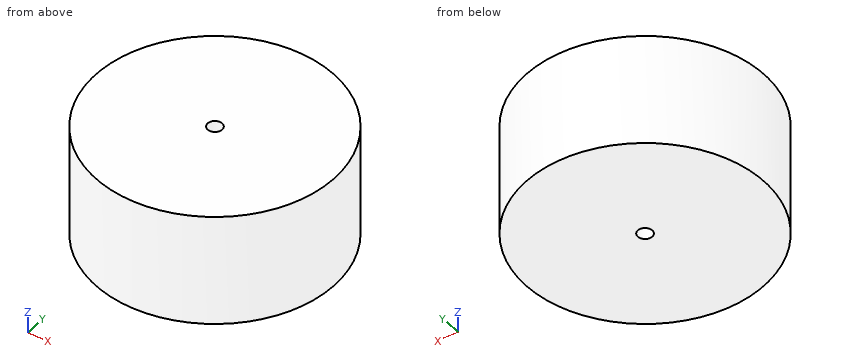
from build123d import *

# Parameters (mm, degrees)
CYLINDER_R     = 3.9
CYLINDER_DEPTH = 60
SKETCH_R       = 64
PAD_DEPTH      = 60


with BuildPart() as cylinder:
    # Cylinder → Cylinder (new body)
    with BuildSketch(Plane.XY):
        Circle(CYLINDER_R)
    extrude(amount=CYLINDER_DEPTH)


with BuildPart() as cut:
    # Sketch → Pad (new body)
    with BuildSketch(Plane.XY):
        Circle(SKETCH_R)
    extrude(amount=PAD_DEPTH)

    # Cut: cut Cylinder
    add(cylinder.part, mode=Mode.SUBTRACT)


with BuildPart() as cut_1:
    # Cut placement: moved
    add(cut.part.moved(Location((-90, -440, 0))))


solid = cut_1.part
Build history of the part. All positions in model axes, mm. Give positions to 0.01 mm unless a question says otherwise; leave off trailing zeros. Loops run counter-clockwise (first coordinate to the right, second up) from the corner with the lowest first, then second, coordinate; pieces in that order, holes last. Notation, with made-up numbers: (-17.5, 58.25) - (9.5, 58.25) arc R19 ccw to (9.5, 81.25) - close; hole circle Ø11 at (16, -4.5). An arc over 180 degrees is marked (long way). Write item = value, one per line. Start each with the question number.
1) Band-saw the part on A-A on x = -90. Give the cut face in (y, z), plus the area to 3 significant figures.
2) Probe probe 1 along Y at (x, z) = (-90, 35.5); probe 2 along Y at (x, z) = (-71.5, 19.5); probe 3 along Y at (x, z) = (-106, 20). List the from-to ranges inside material, lowest first. Write a range as from..to.
3) Drop flat-ended pins along their axis: pin 1 Ø12 at (x, y) = (-83.5, -392.5) entering from -Z; pin 2 Ø6 at (x, z) = (-87.5, 15.5) entering from -Y; pin 3 Ø3 at (y, z) = (-434.5, 9) entering from -X; pin 4 Ø4 at (y, z) = (-468.5, 53) entering from +X. Give the stop position or say it passes through.
4) Band-saw the part on C-C on z = 40. Give the cut face in (x, y).
5) Band-saw the part on B-B on y = -440. Give the cut face in (x, z), plus the area to 3 significant figures.
6) Band-saw the part on D-D on y = -483.5. Give the cut face in (x, z), plus the area to 3 significant figures.
Final values:
q1.outline = (-504, 0) - (-443.9, 0) - (-443.9, 60) - (-504, 60) - close; (-436.1, 0) - (-376, 0) - (-376, 60) - (-436.1, 60) - close
q1.area = 7,210 mm²
q2.probe_1 = -504..-443.9, -436.1..-376
q2.probe_2 = -501.27..-378.73
q2.probe_3 = -501.97..-378.03
q3.pin_1 = 0
q3.pin_2 = -504
q3.pin_3 = -153.87
q3.pin_4 = -31.74
q4.outline = circle Ø128 at (-90, -440); hole circle Ø7.8 at (-90, -440)
q5.outline = (-154, 0) - (-93.9, 0) - (-93.9, 60) - (-154, 60) - close; (-86.1, 0) - (-26, 0) - (-26, 60) - (-86.1, 60) - close
q5.area = 7,210 mm²
q6.outline = (-136.94, 0) - (-43.06, 0) - (-43.06, 60) - (-136.94, 60) - close
q6.area = 5,630 mm²
